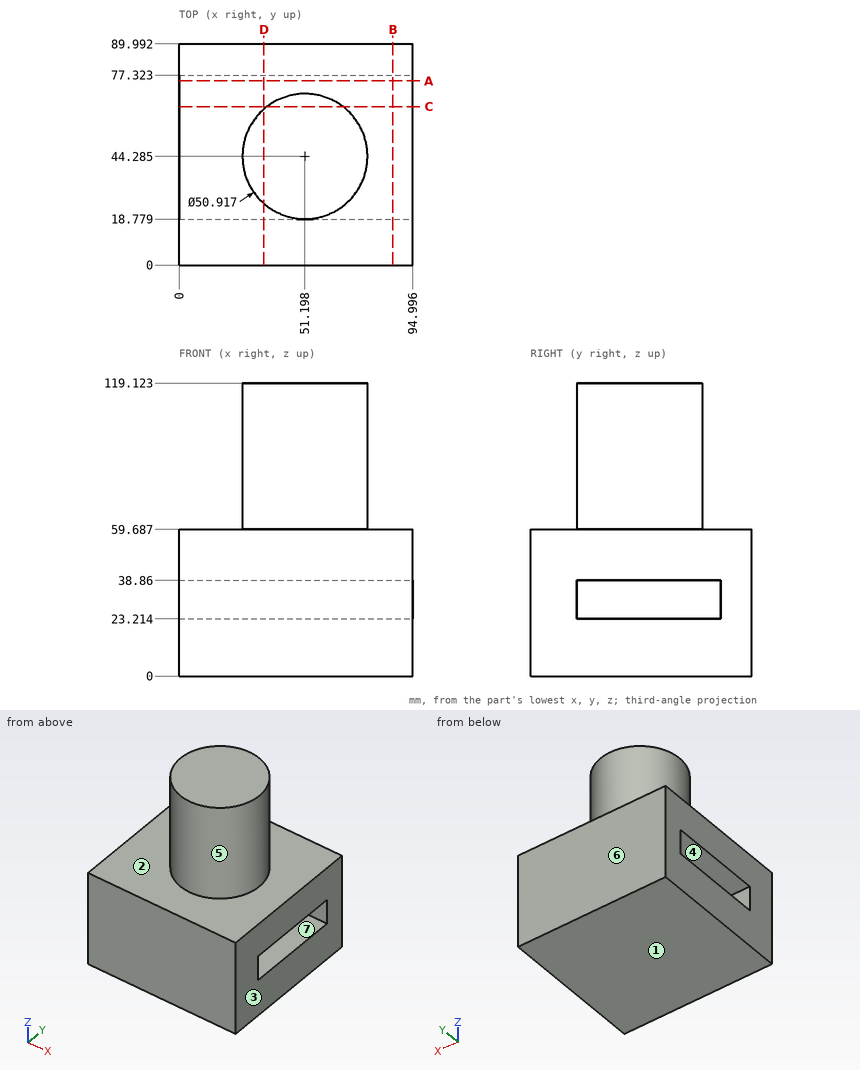
Answer from the drawing. Dimensions are ordinates in mm from the lowest x, y and z of the part. A direction names the side the tool comes from. Round coordinates to 2 decimals unless told otherwise and drop trailing zeros. Write each loop counter-clockwise with the first axis right and the second up, starting at its lowest first coordinate (ties: lowest second). Pieces come first, ordered by that corner, then holes. Notation, with made-up numbers: (-12.75, 71) -> (26.25, 71) arc R8 cw to (26.25, 83) -> close; hole circle Ø6 at (56, -2). An arc over 180 degrees is marked (long way). Answer in a Markdown table with one row per item. Add a question column.
1) Determine the mould class of the marked faces 1, 2, 3 and 4 for opening direction Z: pulls with the +Z half, pulls with the -Z half, needs draft (parallel to the pull), parting line crosses it, or undercut.
2) Consider line 1 (Z direction, x = 60.5, y = 55) (1 decimal); line 2 (Z direction, x = 10.5, y = 39) (1 decimal); line 3 (Y direction, x = 35, z = 36.5). Determine where each line is inside the solid, lowest interval first.
3) Find section C-C, the plane y = 64.5. Determine the outline of the cut face in (x, z) (1 decimal).
4) Given P1, Ø8, axis at x = 41, z = 98, coming from the -Y side; P2, Ø6, axis at x = 24, y = 66.5, coming from the +Z side, each flat-ended and moving along its own axis, determine where each tip first touches the part or whether it passes through.
5) Which of the six approach directions +Z, -Z, +X, -X, +Y, -Y give full straight-line access (tool end or side, diameter ignored) to the marked faces 5, 6 and 7?
6) Find section B-B, the plane x = 87. Determine the outline of the cut face in (y, z) (1 decimal), and give its area (3 significant figures).
7) Find section A-A, the plane y = 75. Determine the outline of the cut face in (x, z) (1 decimal).
8) Find section D-D, the plane x = 34.5. Determine the outline of the cut face in (y, z) (1 decimal).
Findings below:
| question | item | result |
|---|---|---|
| 1 | face 1 | pulls with the -Z half |
| 1 | face 2 | pulls with the +Z half |
| 1 | face 3 | needs draft |
| 1 | face 4 | undercut |
| 2 | line 1 | 0 to 23.2, 38.9 to 119.1 |
| 2 | line 2 | 0 to 23.2, 38.9 to 59.7 |
| 2 | line 3 | 0 to 18.78, 77.32 to 89.99 |
| 3 | outline | (0, 0) -> (95, 0) -> (95, 23.2) -> (0, 23.2) -> close; (0, 38.9) -> (95, 38.9) -> (95, 59.7) -> (66.7, 59.7) -> (66.7, 119.1) -> (35.7, 119.1) -> (35.7, 59.7) -> (0, 59.7) -> close |
| 4 | P1 | y = 19.59 |
| 4 | P2 | z = 59.69 |
| 5 | face 5 | +Z |
| 5 | face 6 | +Z, -Z, +X, -X, +Y |
| 5 | face 7 | +X, -X |
| 6 | outline | (0, 0) -> (90, 0) -> (90, 59.7) -> (0, 59.7) -> close; hole (18.8, 23.2) -> (77.3, 23.2) -> (77.3, 38.9) -> (18.8, 38.9) -> close |
| 6 | area | 4,460 mm² |
| 7 | outline | (0, 0) -> (95, 0) -> (95, 23.2) -> (0, 23.2) -> close; (0, 38.9) -> (95, 38.9) -> (95, 59.7) -> (0, 59.7) -> close |
| 8 | outline | (0, 0) -> (90, 0) -> (90, 59.7) -> (63.5, 59.7) -> (63.5, 119.1) -> (25.1, 119.1) -> (25.1, 59.7) -> (0, 59.7) -> close; hole (18.8, 23.2) -> (77.3, 23.2) -> (77.3, 38.9) -> (18.8, 38.9) -> close |
